Verification items for the finished model (mm, model axes). A direction names the side the tool comes from. Coordinates: 2 decimals unless noted, no trailing zeros. Loops run counter-clockwise (first coordinate to the right, second up) from the corner with the lowest first, then second, coordinate; pieces in that order, holes last.
Q1. Access from +Z, -Z, +X, -X, +Y, -Y to the whole of each face (thin tool, end or side, straight path). Record for faces 1 (the face through (-1.115, -5.865, 1.216)), 2 (the face through (-1, 9, 0)), 3 (the face through (-2.028, -1.676, 3.448)).
Q2. Sectioned sample at C-C (x = 3.5). Enter the section's corners in (y, z), then the cut area to 3 significant figures.
Q3. Material ranges on probe 1 along X at (y, z) = (7.35, 0); probe 2 along X at (y, z) = (9.6, 0); probe 3 along Y at (x, z) = (1.25, 3.5), recorded low to high.
Q4. Go/stop test with flat-tipped pins: P1, Ø1.1, axis at x = 0, z = 0, coming from the +Y side; P2, Ø2, axis at y = -6.5, z = 3, coming from the -X side; P3, Ø1, axis at x = -2.5, y = 1, coming from the +Z side. Record where each tip stops, or that it passes through.
Q5. Sectioned sample at A-A (z = 0). Enter the section's corners in (x, y), then the cut area to 3 significant figures.
Q6. Sectioned sample at D-D (y = 2). Enter the section's corners in (x, z), then the cut area to 3 significant figures.
Q7. Sectioned sample at B-B (y = -2.5). Enter the section's corners in (x, z).
Q8. Mould release check, pull along X, two halves, no side actions. Record for faces 4 (the face through (-1.97, -1.68, -3.48)), 5 (the face through (0, -8.4, -1)), 6 (the face through (2.294, 9.986, 0.509)), 7 (the face through (4, -2, 0)): +X half, -X half, draft (parallel to the pull), parting line (faces both ways), or undercut.
```python
from build123d import *

# Parameters (mm, degrees)
CHAMFER_1_SIZE      = 0.5
CHAMFER_1_SIZE2     = 0.866025404
CUT_EXTRUDE_1_REACH = 15.077
SKETCH_2_R          = 5


with BuildPart() as part:
    # Эскиз1 → Повернуть1 (revolve)
    with BuildSketch(Plane.XY, mode=Mode.PRIVATE) as revolve_1_sk:
        Polygon((2.35, 11), (2.35, 9), (0.5, 9), (0.5, 4), (0, 4), (0, -9.4), (0.85, -9.4), (0.85, -8.4), (1.65, -8.4), (1.65, -3.4), (5, -3.4), (5, 0), (3.15, 0), (3.15, 11), align=None)
    revolve(revolve_1_sk.sketch.rotate(Axis((0, 0, 0), (0, 1, 0)), 90), axis=Axis((0, 0, 0), (0, 1, 0)))

    # Фаска1
    chamfer_1_edges = [part.edges().sort_by_distance(p)[0] for p in [
        (0, 11, 3.15),
    ]]
    chamfer_1_side = [part.faces().sort_by_distance(p)[0] for p in [
        (0, 11, 3.060904546),
    ]]
    chamfer(chamfer_1_edges, length=CHAMFER_1_SIZE, length2=CHAMFER_1_SIZE2, reference=chamfer_1_side[0])

    # Эскиз2 → Вырез-Вытянуть1 (cut, up to next)
    with BuildSketch(Plane(origin=(0, 0, 0), x_dir=(1, 0, 0), z_dir=(0, 1, 0)), mode=Mode.PRIVATE) as cut_extrude_1_sk1:
        Circle(SKETCH_2_R)
        Polygon((-4, 2.309401077), (-4, -2.309401077), (0, -4.618802154), (4, -2.309401077), (4, 2.309401077), (0, 4.618802154), align=None, mode=Mode.SUBTRACT)
    cut_extrude_1_tool1 = extrude(cut_extrude_1_sk1.sketch, amount=-CUT_EXTRUDE_1_REACH, mode=Mode.PRIVATE) & part.part
    add(cut_extrude_1_tool1.solids().sort_by_distance((-4.858579, 0, 0))[0], mode=Mode.SUBTRACT)


solid = part.part
```
Geometry check:
1. face 1: -Y
1. face 2: +Y
1. face 3: +Z, -X, +Y, -Y
2. outline: (-3.4, -2.6) - (0, -2.6) - (0, 2.6) - (-3.4, 2.6) - close
2. area: 17.7 mm2
3. probe 1: x = -3.15 to -0.5, 0.5 to 3.15
3. probe 2: x = -3.15 to -2.35, 2.35 to 3.15
3. probe 3: y = -3.4 to 0
4. P1: stops at y = 9
4. P2: passes through
4. P3: stops at z = 2.43
5. outline: (-4, -3.4) - (-1.65, -3.4) - (-1.65, -8.4) - (-0.85, -8.4) - (-0.85, -9.4) - (0.85, -9.4) - (0.85, -8.4) - (1.65, -8.4) - (1.65, -3.4) - (4, -3.4) - (4, 0) - (3.15, 0) - (3.15, 10.13) - (2.65, 11) - (2.35, 11) - (2.35, 9) - (0.5, 9) - (0.5, 4) - (-0.5, 4) - (-0.5, 9) - (-2.35, 9) - (-2.35, 11) - (-2.65, 11) - (-3.15, 10.13) - (-3.15, 0) - (-4, 0) - close
5. area: 99.9 mm2
6. outline: circle Ø6.3 at (0, 0)
6. area: 31.2 mm2
7. outline: (-4, -2.31) - (0, -4.62) - (4, -2.31) - (4, 2.31) - (0, 4.62) - (-4, 2.31) - close
8. face 4: -X half
8. face 5: draft
8. face 6: undercut
8. face 7: +X half
